from build123d import *

# Parameters (mm, degrees)
SKETCH1_R                       = 22
GEAR_PROFILE_DEPTH              = 10
TEETH_PROFILE_DEPTH             = 37.986484018
TEETH_CIRCULAR_PATTERN_COUNT    = 20
GEAR_BORE_DEPTH                 = 37.770724425
SKETCH4_R                       = 15
SKETCH4_R_2                     = 10
WEIGHT_REDUCTION_POCKET_1_DEPTH = 5


with BuildPart() as part:
    # Sketch1 → Gear Profile (new, symmetric)
    with BuildSketch(Plane.XY):
        Circle(SKETCH1_R)
    extrude(amount=GEAR_PROFILE_DEPTH, both=True)

    # Sketch2 → Teeth Profile (cut, through all)
    with BuildSketch(Plane.XY.offset(10)):
        with BuildLine():
            Line((-0.55092361, 17.5), (0.55092361, 17.5))
            ThreePointArc((0.55092361, 17.5), (1.001895347, 17.692276656), (1.175390804, 18.150801625))
            ThreePointArc((1.175390804, 18.150801625), (1.56580944, 20.17854419), (2.8208, 21.81841166))
            ThreePointArc((2.8208, 21.81841166), (0, 22), (-2.8208, 21.81841166))
            ThreePointArc((-2.8208, 21.81841166), (-1.56580944, 20.17854419), (-1.175390804, 18.150801625))
            ThreePointArc((-1.175390804, 18.150801625), (-1.001895347, 17.692276656), (-0.55092361, 17.5))
        make_face()
    teeth_profile = extrude(amount=-TEETH_PROFILE_DEPTH, mode=Mode.SUBTRACT)

    # Teeth Circular Pattern: Teeth Profile ×20 about axis
    teeth_circular_pattern_axis = Axis((0, 0, 0), (0, 0, 1))
    for i in range(1, TEETH_CIRCULAR_PATTERN_COUNT):
        add(teeth_profile.rotate(teeth_circular_pattern_axis, i * 360 / TEETH_CIRCULAR_PATTERN_COUNT), mode=Mode.SUBTRACT)

    # Sketch3 → Gear Bore (cut, through all)
    with BuildSketch(Plane.XY.offset(10)):
        with BuildLine():
            Line((-0.75, 7.462405778), (-0.75, 8.25))
            Line((-0.75, 8.25), (0.75, 8.25))
            Line((0.75, 8.25), (0.75, 7.462405778))
            ThreePointArc((0.75, 7.462405778), (0, -7.5), (-0.75, 7.462405778))
        make_face()
    extrude(amount=-GEAR_BORE_DEPTH, mode=Mode.SUBTRACT)

    # Sketch4 → Weight reduction pocket 1 (cut)
    with BuildSketch(Plane.XY.offset(10)):
        Circle(SKETCH4_R)
        Circle(SKETCH4_R_2, mode=Mode.SUBTRACT)
    weight_reduction_pocket_1 = extrude(amount=-WEIGHT_REDUCTION_POCKET_1_DEPTH, mode=Mode.SUBTRACT)

    # Weight reduction pocket 2: Weight reduction pocket 1 across plane
    add(weight_reduction_pocket_1.mirror(Plane.XY), mode=Mode.SUBTRACT)


solid = part.part
Geometry: final body of the model. Coordinates: model frame, mm. A direction names the side the tool comes from. Give positions to 0.01 mm unless a question says otherwise; leave off trailing zeros. Loops run counter-clockwise (first coordinate to the right, second up) from the corner with the lowest first, then second, coordinate; pieces in that order, holes last. Notation, with made-up numbers: M 42,78 L 98,78 A35 ccw 98,115 Z; hole C 58,-30 d4. An arc over 180 degrees is marked long. Put each result on its own line as item: value.
1) Cut plane B-B, the plane x = 0. Return the cut outline in (y, z), plus the area to 3 significant figures.
Computed values:
outline: M -17.5,-10 L -15,-10 L -15,-5 L -10,-5 L -10,-10 L -7.5,-10 L -7.5,10 L -10,10 L -10,5 L -15,5 L -15,10 L -17.5,10 Z; M 8.25,-10 L 10,-10 L 10,-5 L 15,-5 L 15,-10 L 17.5,-10 L 17.5,10 L 15,10 L 15,5 L 10,5 L 10,10 L 8.25,10 Z
area: 285 mm^2
2) Mould query, pull axis Y, two halves, no side actions, for faces 5 (the flat face through (2.2, -7.4, 10)), 6 (the cylindrical face through (19.606, 9.98, 0.14)), 7 (the flat face through (-5.4, -16.646, 0.14)), 8 (the cylindrical face through (-4.743, -19.704, 0.14)). Classes: released by +Y, released by -Y, zero draft, split by the parting line, or undercut.
Computed values:
face 5: zero draft
face 6: released by +Y
face 7: released by -Y
face 8: undercut
3) Reachability of faces 1 (the flat face through (0, -17.5, 0)), 2 (the cylindrical face through (-15.419, -13.153, 0.14)), 3 (the flat face through (-5.42, 16.64, 0.14)), 4 (the cylindrical face through (17.27, -10.6, 0.14)) from +Z, -Z, +X, -X, +Y, -Y: full face, straight path, thin tool, end or side. Return the list, or none.
Computed values:
face 1: +Z, -Z, -Y
face 2: +Z, -Z, -X
face 3: +Z, -Z, +Y
face 4: +Z, -Z
4) Cut plane C-C, the plane z = -6.75. Give the number of separate pieces and of enclosed holes in the cut face, plus the area to 3 significant figures.
Computed values:
separate pieces: 2
enclosed holes: 2
area: 667 mm^2
5) First-contact query: P1, Ø0.6, axis at y = 0, z = 2, coming from the +X side; P2, Ø2, axis at x = -6.5, z = 4.5, coming from the +Y side; P3, Ø6, axis at y = 13, z = 5.5, coming from the -X side; P4, Ø12, axis at x = 0, y = 0, coming from the +Z side. Flat tips, straight axial feed; report the tip coordinate or a pass-through.
Computed values:
P1: stops at x = 17.5
P2: stops at y = 18.44
P3: stops at x = -19.6
P4: passes through
6) Cut plane D-D, the plane y = -8.5. Return the cut outline in (x, z).
Computed values:
outline: M -19.39,-10 L -12.36,-10 L -12.36,-5 L -5.27,-5 L -5.27,-10 L 5.27,-10 L 5.27,-5 L 12.36,-5 L 12.36,-10 L 19.39,-10 L 19.39,10 L 12.36,10 L 12.36,5 L 5.27,5 L 5.27,10 L -5.27,10 L -5.27,5 L -12.36,5 L -12.36,10 L -19.39,10 Z
7) Cut plane A-A, the plane y = 0. Return the cut outline in (x, z).
Computed values:
outline: M -17.5,-10 L -15,-10 L -15,-5 L -10,-5 L -10,-10 L -7.5,-10 L -7.5,10 L -10,10 L -10,5 L -15,5 L -15,10 L -17.5,10 Z; M 7.5,-10 L 10,-10 L 10,-5 L 15,-5 L 15,-10 L 17.5,-10 L 17.5,10 L 15,10 L 15,5 L 10,5 L 10,10 L 7.5,10 Z
8) Material intervals for L1, parallel to Y at x = 0, z = -7; L2, parallel to Y at x = 19, z = 7; L3, parallel to X at y = 18.5, z = -1.5, sorted ascending. Write a range as from..to.
Computed values:
L1: y = -17.5..-15, -10..-7.5, 8.25..10, 15..17.5
L2: y = -10.61..-8.02, -4.77..-1.22, 1.22..4.77, 8.02..10.61
L3: x = -10.68..-7.55, -4.72..-1.17, 1.17..4.72, 7.55..10.68
